Input: dimensioned drawing with shaded views. Units: mm. Origin: part minimum x, y, z. A direction names the side the tool comes from. Coordinates: 2 decimals unless noted, no trailing zeros. Order: outer loops, then holes, each group sorted by start corner. A loop starts at its lowest first (then second) coordinate and runs counter-clockwise, first axis right, second up. Notation, with made-up numbers: (40, 52) -> (68, 52) arc R32 ccw to (68, 91) -> close; hole circle Ø2 at (-35, 34.25). An arc over 180 degrees is marked (long way). Put each result on its own line as item: value.
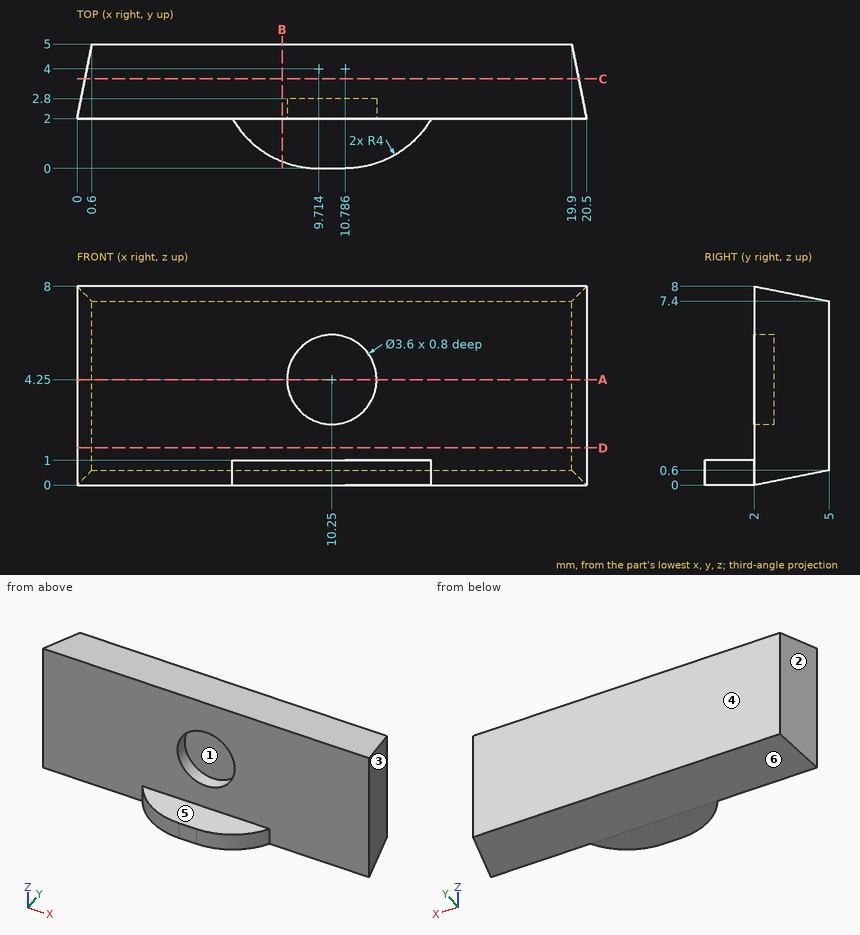
1. Set-up query: the marked faces 5 and 6. Return all of +Z, -Z, +X, -X, +Y, -Y with unobstructed straight access to the full face (end or side cutting, diameter ignored); none if empty.
Numbers:
face 5: +Z, +X, -X, -Y
face 6: -Z, +X, -X, +Y
2. Cut plane C-C on y = 3.6. Output: boundary loops of the cut face in (x, z).
Numbers:
outline: (0.32, 0.32) -> (20.18, 0.32) -> (20.18, 7.68) -> (0.32, 7.68) -> close
3. Cut plane D-D on z = 1.5. Output: boundary loops of the cut face in (x, y), plus the area to 3 significant figures.
Numbers:
outline: (0, 2) -> (20.5, 2) -> (19.9, 5) -> (0.6, 5) -> close
area: 59.7 mm2
4. Cut plane B-B on x = 8.25. Output: boundary loops of the cut face in (y, z).
Numbers:
outline: (0.28, 0) -> (2, 0) -> (5, 0.6) -> (5, 7.4) -> (2, 8) -> (2, 1) -> (0.28, 1) -> close
5. Ray query, line 1 along X through (y, z) = (2.55, 4.25); line 2 along Y through (x, z) = (1.75, 1.5); line 3 along Z through (x, y) = (8.25, 0.65). Return the intervals inside material, ascending.
Numbers:
line 1: x = 0.11 to 8.45, 12.05 to 20.39
line 2: y = 2 to 5
line 3: z = 0 to 1
6. Pull-direction query (X, two-part tool) for the marked faces 1, 2, 3 and 4; classes: pulls with the +X half, pulls with the -X half, needs draft (parallel to the pull), parting line crosses it, or undercut.
Numbers:
face 1: undercut
face 2: pulls with the -X half
face 3: pulls with the +X half
face 4: needs draft
7. First-contact query: pin 1 (3 mm diameter, centred on x = 14, z = 4.5, fed in from -Y); pin 2 (1 mm diameter, centred on x = 11, y = 0.5, fed in from +Z); pin 3 (1.1 mm diameter, centred on x = 11, z = 3.5, fed in from -Y). Flat tips, straight axial feed; report the tip coordinate or a pass-through.
Numbers:
pin 1: stops at y = 2
pin 2: stops at z = 1
pin 3: stops at y = 2.8
8. Cut plane A-A on z = 4.25. Output: boundary loops of the cut face in (x, y).
Numbers:
outline: (0, 2) -> (8.45, 2) -> (8.45, 2.8) -> (12.05, 2.8) -> (12.05, 2) -> (20.5, 2) -> (19.9, 5) -> (0.6, 5) -> close
